The model under review builds one solid part; all positions refer to its coordinate system, in mm. A direction names the side the tool comes from. Round coordinates to 2 decimals unless told otherwise and drop trailing zeros. Write each loop counter-clockwise with the first axis right and the second up, starting at its lowest first coordinate (ties: lowest second). Pieces come first, ordered by that corner, then holes.
Item 1: To check wall thickness, follow L1, parallel to X at y = 1.75, z = 5.5; L2, parallel to Z at x = -17, y = 3.1; L3, parallel to Z at x = -15.5, y = 0.4. State the ranges of each line that lie inside material, in increasing order.
Item 2: Draft analysis for pull direction Z (two halves, no side actions). For faces 3 (the face through (25, 3, 0)), 4 (the face through (-23.289, 2.958, 38.196)), 5 (the face through (-17, 3, 2.032)), state which applies: +Z half, -Z half, draft (parallel to the pull), parting line (faces both ways), or undercut.
Item 3: Add section A-A (z = -30). Give the boundary of the cut face in (x, y), plus the area to 3 significant figures.
Item 4: Add section C-C (z = 7.5). Give the boundary of the cut face in (x, y), plus the area to 3 significant figures.
Item 5: Clearance check with a flat-ended pin moving along its axis: pin 1 Ø3.5 at (x, z) = (16, -4) entering from -Y. State where the tip first meets the part, or that it passes through.
Item 6: Machinability: for faces 1 (the face through (18.55, 2.96, -29.94)), 2 (the face through (0, 0, -1)), which of the approach directions +Z, -Z, +X, -X, +Y, -Y give a long, thin tool a straight path to every point of the face, cutting with its end or side? Answer none if there is none.
Item 7: Add section B-B (x = -16.55). Give the boundary of the cut face in (y, z).
Item 8: Add section D-D (y = 3.4). State how many separate pieces and enclosed holes the cut face has, plus the area to 3 significant figures.
```python
from build123d import *

# Parameters (mm, degrees)
EXTRUDE_1_DEPTH      = 6
SKETCH_2_R           = 2.55
CUT_EXTRUDE_1_DEPTH  = 7
CUT_EXTRUDE_2_DEPTH  = 7
SKETCH_31_R          = 2.1
SKETCH_31_W          = 7
SKETCH_31_H          = 6
CUT_EXTRUDE_11_DEPTH = 7
SKETCH_32_R          = 2.1
SKETCH_32_W          = 7
SKETCH_32_H          = 6
CUT_EXTRUDE_12_DEPTH = 7


with BuildPart() as part:
    # Эскиз1 → Бобышка-Вытянуть1 (new body)
    with BuildSketch(Plane(origin=(0, 0, 0), x_dir=(1, 0, 0), z_dir=(0, 1, 0))):
        with BuildLine():
            Line((-19, -40), (19, -40))
            ThreePointArc((19, -40), (23.242640687, -38.242640687), (25, -34))
            Line((25, -34), (25, 34))
            ThreePointArc((25, 34), (23.242640687, 38.242640687), (19, 40))
            Line((19, 40), (-19, 40))
            ThreePointArc((-19, 40), (-23.242640687, 38.242640687), (-25, 34))
            Line((-25, 34), (-25, -34))
            ThreePointArc((-25, -34), (-23.242640687, -38.242640687), (-19, -40))
        make_face()
    extrude(amount=EXTRUDE_1_DEPTH)

    # Эскиз2 → Вырез-Вытянуть1 (cut, through all)
    with BuildSketch(Plane.XZ):
        with Locations((-17, -30)):
            Circle(SKETCH_2_R)
        with Locations((-17, 30)):
            Circle(SKETCH_2_R)
        with BuildLine():
            Line((16, -32.55), (14, -32.55))
            ThreePointArc((14, -32.55), (11.45, -30), (14, -27.45))
            Line((14, -27.45), (16, -27.45))
            ThreePointArc((16, -27.45), (18.55, -30), (16, -32.55))
        make_face()
        with BuildLine():
            Line((16, 32.55), (14, 32.55))
            ThreePointArc((14, 32.55), (11.45, 30), (14, 27.45))
            Line((14, 27.45), (16, 27.45))
            ThreePointArc((16, 27.45), (18.55, 30), (16, 32.55))
        make_face()
    extrude(amount=-CUT_EXTRUDE_1_DEPTH, mode=Mode.SUBTRACT)

    # Эскиз3 → Вырез-Вытянуть2 (cut, through all)
    with BuildSketch(Plane.XZ):
        with BuildLine():
            Line((-25, -2), (-25, 2))
            ThreePointArc((-25, 2), (-24.414213562, 0.585786438), (-23, 0))
            ThreePointArc((-23, 0), (-24.414213562, -0.585786438), (-25, -2))
        make_face()
    extrude(amount=-CUT_EXTRUDE_2_DEPTH, mode=Mode.SUBTRACT)

    # Эскиз31 → Вырез-Вытянуть11 (cut, through all)
    with BuildSketch(Plane(origin=(30.45, 0, -4), x_dir=(0, 0, 1), z_dir=(0, -1, 0))):
        with Locations((0, 47)):
            Circle(SKETCH_31_R)
        with Locations((9.531849908, 47)):
            Rectangle(SKETCH_31_W, SKETCH_31_H)
        with Locations((-9.531849908, 47)):
            Rectangle(SKETCH_31_W, SKETCH_31_H)
    extrude(amount=-CUT_EXTRUDE_11_DEPTH, mode=Mode.SUBTRACT)

    # Эскиз32 → Вырез-Вытянуть12 (cut, through all)
    with BuildSketch(Plane(origin=(-31, 0, -4), x_dir=(0, 0, -1), z_dir=(0, -1, 0))):
        with Locations((0, 47)):
            Circle(SKETCH_32_R)
        with Locations((9.531849908, 47)):
            Rectangle(SKETCH_32_W, SKETCH_32_H)
        with Locations((-9.531849908, 47)):
            Rectangle(SKETCH_32_W, SKETCH_32_H)
    extrude(amount=-CUT_EXTRUDE_12_DEPTH, mode=Mode.SUBTRACT)


solid = part.part
```
Numbers:
1. L1: x = -25 to -19.55, -13.55 to 13, 19 to 25
1. L2: z = -40 to -32.55, -27.45 to -17.03, -10.03 to -6.05, -1.95 to 2.03, 9.03 to 27.45, 32.55 to 40
1. L3: z = -40 to -32.06, -27.94 to -17.03, -10.03 to -5.82, -2.18 to 2.03, 9.03 to 27.94, 32.06 to 40
2. face 3: draft
2. face 4: +Z half
2. face 5: undercut
3. outline: (-25, 0) - (-19.55, 0) - (-19.55, 6) - (-25, 6) - close; (-14.45, 0) - (11.45, 0) - (11.45, 6) - (-14.45, 6) - close; (18.55, 0) - (25, 0) - (25, 6) - (18.55, 6) - close
3. area: 227 mm2
4. outline: (-25, 0) - (-19.55, 0) - (-19.55, 6) - (-25, 6) - close; (-13.55, 0) - (13, 0) - (13, 6) - (-13.55, 6) - close; (19, 0) - (25, 0) - (25, 6) - (19, 6) - close
4. area: 228 mm2
5. pin 1: passes through
6. face 1: +Y, -Y
6. face 2: +Z, -Z, +X, -X, -Y
7. outline: (0, -40) - (6, -40) - (6, -32.51) - (0, -32.51) - close; (0, -27.49) - (6, -27.49) - (6, -17.03) - (0, -17.03) - close; (0, -10.03) - (6, -10.03) - (6, -6.1) - (0, -6.1) - close; (0, -1.9) - (6, -1.9) - (6, 2.03) - (0, 2.03) - close; (0, 9.03) - (6, 9.03) - (6, 27.49) - (0, 27.49) - close; (0, 32.51) - (6, 32.51) - (6, 40) - (0, 40) - close
8. separate pieces: 1
8. enclosed holes: 10
8. area: 3,670 mm2
